Print and shaded views of the part. All mm, measured from the part's lowest x, y and z. A direction names the side the tool comes from. Round coordinates to 2 decimals unless told otherwise and drop trailing zeros. Order: outer loops, then holes, each group sorted by start corner. A loop starts at its lowest first (then second) coordinate and runs counter-clockwise, first axis right, second up. Notation, with made-up numbers: (-32, 69) - (-16, 69) arc R22 cw to (-16, 102) - close; hole circle Ø11 at (-19.75, 34). An arc over 180 degrees is marked (long way). Write item = value, one per line.
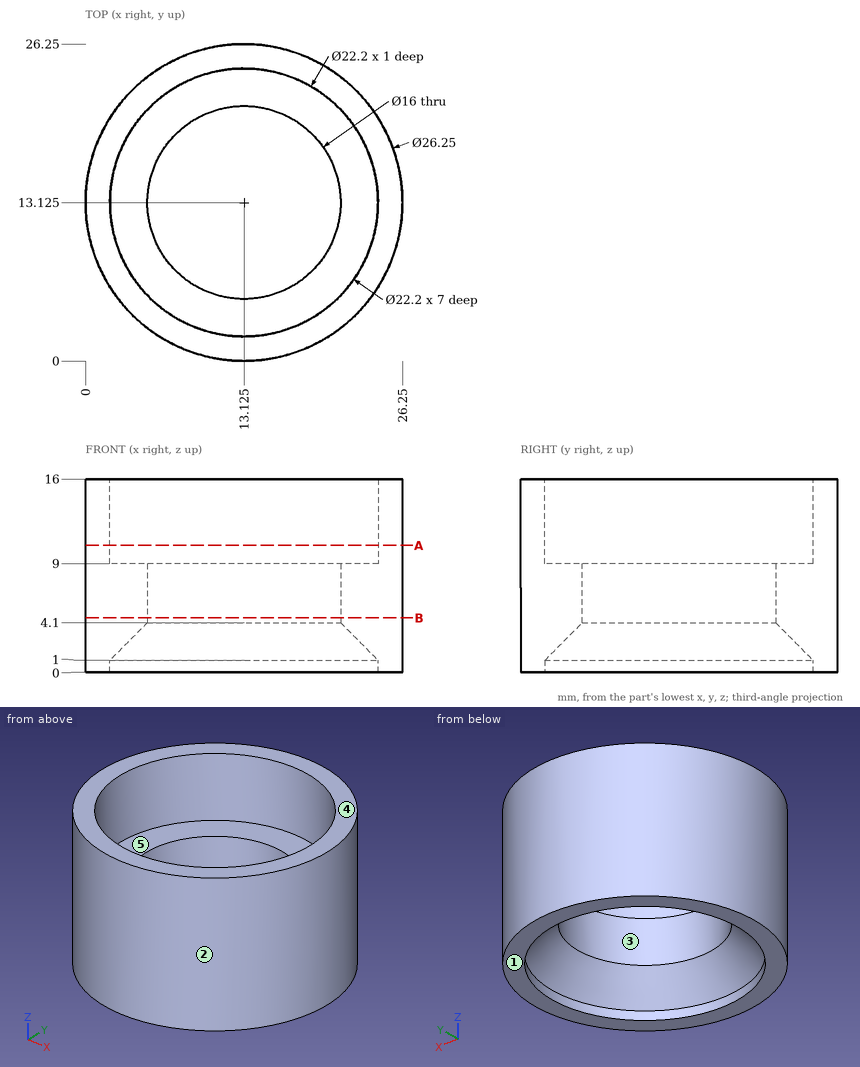
(1) Probe line 1 along Y through (x, z) = (16.25, 1); line 2 along Y through (x, z) = (21, 10.5) (3 decimals); line 3 along X through (y, z) = (17.25, 9.75). List the from-to ranges inside material, lowest first.
Solved:
line_1 = 0.38 to 2.47, 23.78 to 25.87
line_2 = 2.625 to 5.302, 20.948 to 23.625
line_3 = 0.67 to 2.82, 23.43 to 25.58
(2) Drop flat-ended pins along their axis: pin 1 (10 mm diameter, centred on x = 18.5, y = 15.5, fed in from +Z); pin 2 (3 mm diameter, centred on x = 20.5, z = 6.5, fed in from -Y); pin 3 (1 mm diameter, centred on x = 16.5, z = 5, fed in from +Y). Give the stop position or say it passes through.
Solved:
pin_1 = 9
pin_2 = 1.39
pin_3 = 25.93
(3) Band-saw the part on B-B on z = 4.5. List the corners of the cut face in (x, y) (3 decimals), plus the area to 3 significant figures.
Solved:
outline = circle Ø26.25 at (13.125, 13.125); hole circle Ø16 at (13.125, 13.125)
area = 340 mm²
(4) Tool access for the marked faces 4 and 5: list every direction of +Z, -Z, +X, -X, +Y, -Y with a clear straight run to the whole face (end or side of a thin tool).
Solved:
face_4 = +Z, +X, -X, +Y, -Y
face_5 = +Z
(5) Band-saw the part on A-A on z = 10.5. List the corners of the cut face in (x, y) (3 decimals), plus the area to 3 significant figures.
Solved:
outline = circle Ø26.25 at (13.125, 13.125); hole circle Ø22.2 at (13.125, 13.125)
area = 154 mm²
(6) Pull direction X, two halves, no side cores. Call the marked faces 1, 2 and 3: released by +X, released by -X, zero draft, split by the parting line, or undercut.
Solved:
face_1 = zero draft
face_2 = split by the parting line
face_3 = undercut
